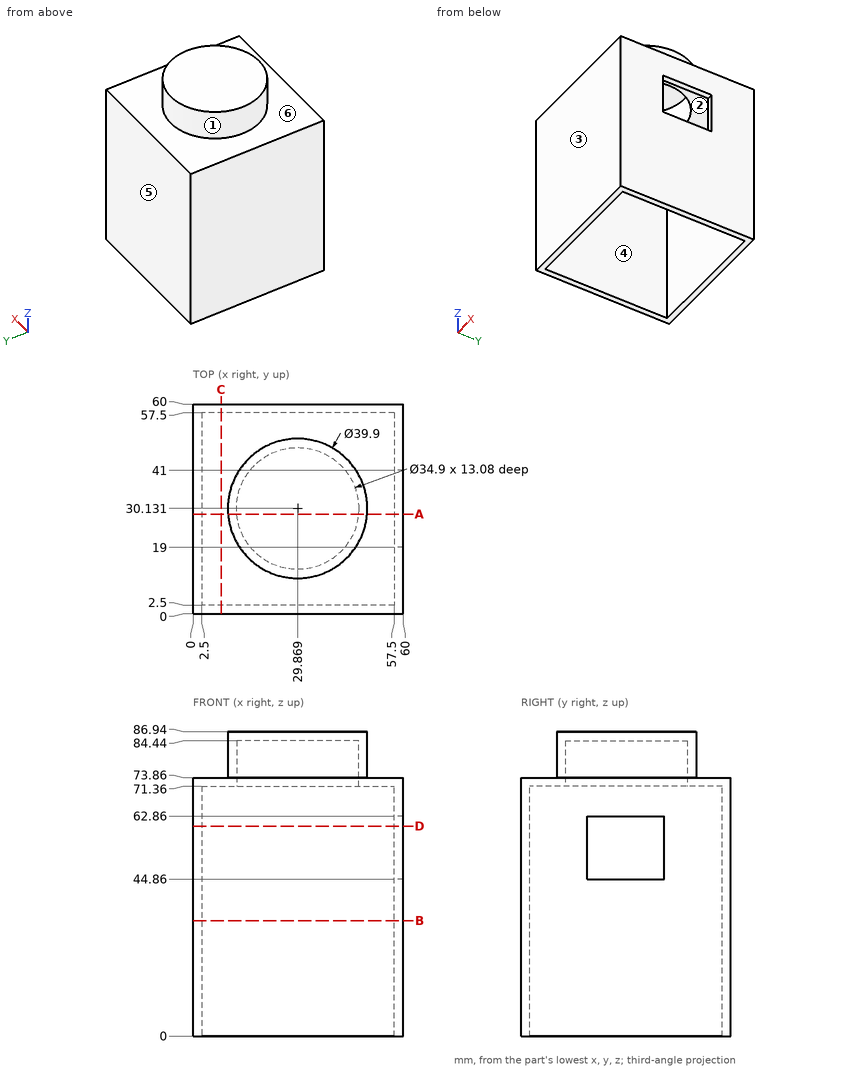
Geometry check sheet. Reference: drawing and pictorial views, mm from the part's lowest x, y, z. A direction names the side the tool comes from. Coordinates: 2 decimals unless noted, no trailing zeros. Order: outer loops, then holes, each group sorted by start corner. A loop starts at its lowest first (then second) coordinate and runs counter-clockwise, first axis right, second up. Notation, with made-up numbers: (89, 72) - (133, 72) arc R36 cw to (133, 108) - close; hole circle Ø7 at (-40, 88). An arc over 180 degrees is marked (long way). Answer in a Markdown table with one row per item. Add a question column.
1) Cross-section at B-B, the plane z = 33. Record the cut outline in (x, y).
2) Material ranges on line 1 along Y through (x, z) = (22.5, 48); line 2 along X through (y, z) = (39, 55.5), recorded low to high. Write a range as [from, to].
3) Cross-section at D-D, the plane z = 60. Record the cut outline in (x, y).
4) Release check for a two-part mould opening along Y. For the marked faces 4, 5 and 6 record: +Y half, -Y half, draft (parallel to the pull), parting line (faces both ways), or undercut.
5) Cross-section at A-A, the plane y = 28.5. Record the cut outline in (x, z).
6) Set-up check for the marked faces 1, 2 and 3: record each of +Z, -Z, +X, -X, +Y, -Y from which the full face is reachable in a straight line by a thin tool's end or side.
7) Gauge pin test, flat ends, axial feed: P1, Ø4, axis at x = 47, y = 52.5, coming from the +Z side; P2, Ø8, axis at x = 45, y = 35.5, coming from the -Z side; P3, Ø1, axis at y = 24, z = 12.5, coming from the -X side; P4, Ø17.5, axis at x = 37.5, y = 29.5, coming from the -Z side. Record the tip position at first contact, or that the pin passes through.
8) Cross-section at C-C, the plane x = 8. Record the cut outline in (y, z).
Check result:
| question | item | result |
|---|---|---|
| 1 | outline | (0, 0) - (60, 0) - (60, 60) - (0, 60) - close; hole (2.5, 2.5) - (57.5, 2.5) - (57.5, 57.5) - (2.5, 57.5) - close |
| 2 | line 1 | y = [0, 2.5], [57.5, 60] |
| 2 | line 2 | x = [0, 2.5] |
| 3 | outline | (0, 0) - (60, 0) - (60, 19) - (57.5, 19) - (57.5, 2.5) - (2.5, 2.5) - (2.5, 57.5) - (57.5, 57.5) - (57.5, 41) - (60, 41) - (60, 60) - (0, 60) - close |
| 4 | face 4 | undercut |
| 4 | face 5 | +Y half |
| 4 | face 6 | draft |
| 5 | outline | (0, 0) - (2.5, 0) - (2.5, 71.36) - (12.5, 71.36) - (12.5, 84.44) - (47.24, 84.44) - (47.24, 71.36) - (57.5, 71.36) - (57.5, 62.86) - (60, 62.86) - (60, 73.86) - (49.75, 73.86) - (49.75, 86.94) - (9.99, 86.94) - (9.99, 73.86) - (0, 73.86) - close; (57.5, 0) - (60, 0) - (60, 44.86) - (57.5, 44.86) - close |
| 6 | face 1 | +Z |
| 6 | face 2 | -Z |
| 6 | face 3 | +Z, -Z, +X, -X, -Y |
| 7 | P1 | stops at z = 73.86 |
| 7 | P2 | stops at z = 71.36 |
| 7 | P3 | stops at x = 0 |
| 7 | P4 | stops at z = 84.44 |
| 8 | outline | (0, 0) - (2.5, 0) - (2.5, 71.36) - (57.5, 71.36) - (57.5, 0) - (60, 0) - (60, 73.86) - (0, 73.86) - close |
